Can you work these out from the model? Positions are in its coordinate system, mm. A direction names the side the tool comes from. Coordinates: 2 decimals unless noted, no trailing zeros. Order: outer loops, then holes, each group sorted by start corner. A loop starts at its lowest first (then second) coordinate and runs counter-clockwise, first axis right, second up. Notation, with made-up numbers: (21, -36.75) -> (48, -36.75) arc R8 ccw to (48, -21.75) -> close; hole circle Ø5 at (83.5, -4.5). An arc over 180 degrees is marked (long way). Answer in a Markdown table with one row per item. Add a question column.
1. Imagine slicing it at A-A on x = -25.4. Write out the boundary of the cut face in (y, z).
2. If I drill on line 1 along X through (y, z) = (40.5, 15.5); line 2 along Z through (x, y) = (-92, 5), over which ranges is the centre line in solid material (lowest first)? Write a range as [from, to].
3. We'd pull the mould along X, two halves only. Please class faces 3 (the face through (-94.737, -2.623, 17.798)), 4 (the face through (-5.65, -0.69, 17.8)), 5 (the face through (11, -12, 19.05)), 6 (the face through (-127, -14, 9)): pulls with the +X half, pulls with the -X half, needs draft (parallel to the pull), parting line crosses it, or undercut.
4. On a 3-axis mill with a long thin cutter (end or side, diameter ignored), from which of +Z, -Z, +X, -X, +Y, -Y can I reach the whole of each face in a straight line? I mean faces 1 (the face through (-88, 1, 16.51)), 2 (the face through (144.876, -68.07, 9.392)). Say none if no direction works.
5. Will these pins go through, and if not, where does the flat tip stop? pin 1 (3.5 mm diameter, centred on x = -25, y = 9.5, fed in from +Z); pin 2 (8.5 mm diameter, centred on x = -118.03, y = -68.37, fed in from -Z).
Autodesk Inventor part; units mm, degrees
ref_plane "YZ Plane" through (0, 0, 0) normal (1, 0, 0) x (0, 1, 0)
ref_plane "XZ Plane" through (0, 0, 0) normal (0, 1, 0) x (-1, 0, 0)
ref_plane "XY Plane" through (0, 0, 0) normal (0, 0, 1) x (1, 0, 0)
sketch "Sketch1" plane through (0, 0, 0) normal (0, 0, 1) x (1, 0, 0)
  line L0 (-127, 50.8) -> (152.4, 50.8)
  line L1 (152.4, 50.8) -> (152.4, -76.2)
  line L2 (152.4, -76.2) -> (-127, -76.2)
  line L3 (-127, -76.2) -> (-127, 50.8)
  point P0 (0, 0)
  dimension "d0" = 127
  dimension "d1" = 279.4
extrude "Extrusion1" add sketch "Sketch1" along normal blind 19.05
sketch "Sketch2" plane through (0, 0, 19.05) normal (0, 0, 1) x (1, 0, 0)
  arc A0 (-73.0244, 15.878) -> (-73.0246, -22.228) centre (-75.5284, -3.175) ccw
  arc A1 (-73.1475, 9.5485) -> (-73.025, -15.875) centre (-75.5284, -3.175) ccw
  arc A2 (-73.1475, 9.5485) -> (-73.0244, 15.878) centre (-72.5572, 12.703) ccw
  arc A3 (-73.2146, -22.252) -> (-73.025, -15.875) centre (-73.603, -19.0491) ccw
  line L0 (-61.1063, -15.875) -> (-61.1063, 9.5485)
  arc A4 (-61.1063, -15.875) -> (-53.975, -15.875) centre (-57.5407, -16.9375) ccw
  arc A5 (-53.975, 9.5485) -> (-61.1063, 9.5485) centre (-57.5407, 10.5766) ccw
  line L1 (-53.975, 9.5485) -> (-53.975, -9.525)
  arc A6 (-38.1, -9.525) -> (-53.975, -9.525) centre (-46.0375, -11.2959) ccw
  line L2 (-38.1, -9.525) -> (-38.1, -17.8441)
  arc A7 (-44.6048, -17.106) -> (-38.1, -17.8441) centre (-41.3943, -17.8441) ccw
  arc A8 (-44.6048, -17.106) -> (-53.975, -15.875) centre (-49.231, -16.0424) ccw
  circle A9 centre (-25.4, 9.5485) radius 3.4758
  arc A10 (-28.8758, -16.0424) -> (-21.9242, -16.0424) centre (-25.4, -17.3897) ccw
  arc A11 (-21.9242, -3.1632) -> (-28.8758, -3.1632) centre (-25.4, -2.0594) ccw
  line L3 (-28.8758, -3.1632) -> (-28.8758, -16.0424)
  line L4 (-21.9242, -3.1632) -> (-21.9242, -16.0424)
  arc A12 (-12.6126, -16.1823) -> (-6.2626, -16.1823) centre (-9.4376, -17.7266) ccw
  line L5 (-12.6126, -16.1823) -> (-12.6126, -0.1511)
  arc A13 (6.1684, -2.399) -> (-12.6126, -0.1511) centre (-3.0876, -0.1511) ccw
  line L6 (-6.2626, -16.1823) -> (-6.2626, -6.4899)
  arc A14 (0, 0) -> (6.1684, -2.399) centre (2.9241, -1.6111) ccw
  arc A15 (0, 0) -> (-6.2626, -6.4899) centre (-2.3813, -3.9688) ccw
  circle A16 centre (22.4437, -5.0591) radius 11.2637
  circle A17 centre (22.4437, -5.0591) radius 5.6341
  line L7 (28.0778, -14.8125) -> (28.0778, -19.8605)
  line L8 (32.1971, -10.6931) -> (32.1971, -19.8605)
  arc A18 (28.0778, -19.8605) -> (32.1971, -19.8605) centre (30.1375, -19.8605) ccw
  circle A19 centre (54.7585, -2.6676) radius 11.4369
  circle A20 centre (54.7585, -2.6676) radius 6.4193
  arc A21 (43.3216, -19.5287) -> (64.2241, -9.0869) centre (51.9093, -10.5775) ccw
  arc A22 (43.3216, -19.5287) -> (40.471, -26.1835) centre (41.8963, -22.8561) ccw
  arc A23 (40.471, -26.1835) -> (66.1955, -2.6676) centre (50.4992, -11.3254) ccw
emboss "Emboss1" sketch "Sketch2" operation cut depth 2.54 direction (0, 0, -1)
hole "Hole1" at (-116.218, 41.2565, 19.05) direction (0, 0, -1) diameter 6.35 end through all
hole "Hole2" at (-118.0348, -68.3727, 19.05) direction (0, 0, -1) diameter 6.35 end through all
hole "Hole3" at (138.1431, 40.9115, 19.05) direction (0, 0, -1) diameter 6.35 end through all
hole "Hole4" at (141.7768, -68.7579, 19.05) direction (0, 0, -1) diameter 6.35 end through all
properties part number "NameTag"
Answers follow:
| question | item | result |
|---|---|---|
| 1 | outline | (-76.2, 0) -> (50.8, 0) -> (50.8, 19.05) -> (13.02, 19.05) -> (13.02, 16.51) -> (6.07, 16.51) -> (6.07, 19.05) -> (1.59, 19.05) -> (1.59, 16.51) -> (-21.12, 16.51) -> (-21.12, 19.05) -> (-76.2, 19.05) -> close |
| 2 | line 1 | x = [-127, -119.3], [-113.13, 134.99], [141.29, 152.4] |
| 2 | line 2 | z = [0, 16.51] |
| 3 | face 3 | undercut |
| 3 | face 4 | undercut |
| 3 | face 5 | needs draft |
| 3 | face 6 | pulls with the -X half |
| 4 | face 1 | +Z |
| 4 | face 2 | +Z, -Z |
| 5 | pin 1 | stops at z = 16.51 |
| 5 | pin 2 | stops at z = 0 |
